CAD build for the part. Positions are in the model's coordinates, mm. Face numbers are marked on the shaded views. A direction names the side the tool comes from. Round coordinates to 2 decimals unless told otherwise and drop trailing zeros. Loops run counter-clockwise (first coordinate to the right, second up) from the corner with the lowest first, then second, coordinate; pieces in that order, holes last. Notation, with made-up numbers: M 44,-4 L 92,-4 A20 ccw 92,21 Z; hole C -7.75,19.5 d2. An arc over 180 degrees is marked long. Use one line per item in the form item = value.
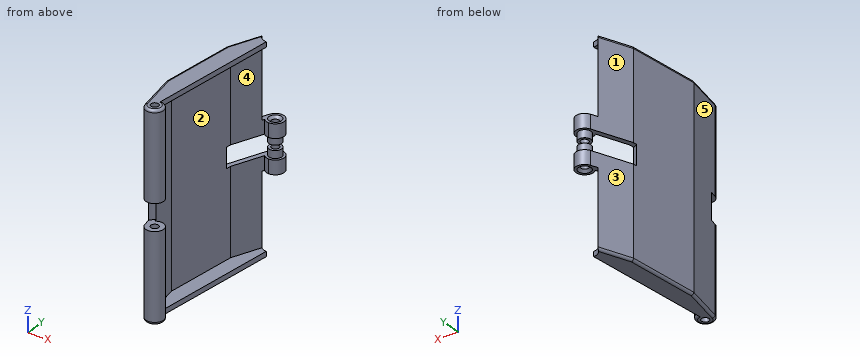
from build123d import *
from build123d.topology import SkipClean

# Parameters (mm, degrees)
CROQUIS2_R              = 1.5
SALIENTE_EXTRUIR1_DEPTH = 40
CORTAR_EXTRUIR8_DEPTH   = 38
CROQUIS21_R             = 4.5
CORTAR_EXTRUIR9_DEPTH   = 30.5
CHAFL_N1_SIZE           = 1
CROQUIS22_R             = 18.418021377
CORTAR_EXTRUIR10_DEPTH  = 4
SALIENTE_EXTRUIR2_START = 3
CROQUIS23_R             = 2.5
CROQUIS23_R_2           = 1.5
SALIENTE_EXTRUIR2_DEPTH = 3
CROQUIS24_R             = 4.5
CORTAR_EXTRUIR11_DEPTH  = 5.2
REDONDEO_CABLE_PLANO_R  = 1


with BuildPart() as part:
    # Croquis2 → Saliente-Extruir1 (new body)
    with BuildSketch(Plane.XY):
        with BuildLine():
            Line((-81.260569926, 30.810305605), (-87.479685276, 15.380704046))
            Line((-87.479685276, 15.380704046), (-90.491189661, -14.467760593))
            Line((-90.491189661, -14.467760593), (-87.479519283, -30.828684819))
            ThreePointArc((-87.479519283, -30.828684819), (-81.463725094, -32.56707429), (-83.686009105, -26.712739874))
            Line((-83.686009105, -26.712739874), (-78.365684691, 26.019547656))
            ThreePointArc((-78.365684691, 26.019547656), (-75.018767914, 31.311988091), (-81.260569926, 30.810305605))
        make_face()
        with Locations((-78.014342512, 29.50186853)):
            Circle(CROQUIS2_R, mode=Mode.SUBTRACT)
        with Locations((-84.037351283, -30.195060749)):
            Circle(CROQUIS2_R, mode=Mode.SUBTRACT)
    extrude(amount=SALIENTE_EXTRUIR1_DEPTH)

    # Croquis20 → Cortar-Extruir8 (cut)
    with BuildSketch(Plane(origin=(0, 0, 0), x_dir=(-1, 0, 0), z_dir=(0, 0, -1))):
        with BuildLine():
            Line((80.58776607, 27.129635154), (85.518345507, 14.896886302))
            Line((85.518345507, 14.896886302), (88.472734145, -14.385476766))
            Line((88.472734145, -14.385476766), (86.085050495, -27.356587931))
            ThreePointArc((86.085050495, -27.356587931), (84.944567837, -26.814682349), (83.686009105, -26.712739874))
            Line((83.686009105, -26.712739874), (78.365684691, 26.019547656))
            ThreePointArc((78.365684691, 26.019547656), (79.578515526, 26.370836307), (80.58776607, 27.129635154))
        make_face()
    extrude(amount=-CORTAR_EXTRUIR8_DEPTH, mode=Mode.SUBTRACT)

    # Croquis21 → Cortar-Extruir9 (cut)
    with BuildSketch(Plane.XY.offset(40)):
        with Locations((-78.014342512, 29.50186853)):
            Circle(CROQUIS21_R)
    extrude(amount=-CORTAR_EXTRUIR9_DEPTH, mode=Mode.SUBTRACT)

    # Chaflán1
    chafl_n1_edges = [part.edges().sort_by_distance(p)[0] for p in [
        (-79.514342512, 29.50186853, 9.5),
    ]]
    chamfer(chafl_n1_edges, length=CHAFL_N1_SIZE)

    # Croquis22 → Cortar-Extruir10 (cut)
    with BuildSketch(Plane(origin=(0, 0, 0), x_dir=(-1, 0, 0), z_dir=(0, 0, -1))):
        with Locations((78.014342512, 29.50186853)):
            Circle(CROQUIS22_R)
    extrude(amount=-CORTAR_EXTRUIR10_DEPTH, mode=Mode.SUBTRACT)

    # Croquis23 → Saliente-Extruir2 (add)
    with SkipClean():  # the faces are left unmerged after this step: merging them gives an invalid solid
        with BuildSketch(Plane(origin=(0, 0, 4), x_dir=(-1, 0, 0), z_dir=(0, 0, -1)).offset(SALIENTE_EXTRUIR2_START)):
            with Locations((78.014342512, 29.50186853)):
                Circle(CROQUIS23_R)
            with Locations((78.014342512, 29.50186853)):
                Circle(CROQUIS23_R_2, mode=Mode.SUBTRACT)
        extrude(amount=-SALIENTE_EXTRUIR2_DEPTH)

    # Croquis24 → Cortar-Extruir11 (cut)
    with SkipClean():  # the faces are left unmerged after this step: merging them gives an invalid solid
        with BuildSketch(Plane(origin=(0, 0, 0), x_dir=(-1, 0, 0), z_dir=(0, 0, -1))):
            with Locations((84.037351283, -30.195060749)):
                Circle(CROQUIS24_R)
        extrude(amount=-CORTAR_EXTRUIR11_DEPTH, mode=Mode.SUBTRACT)

    # Simetría1: part across plane


with BuildPart() as part_1:
    with SkipClean():  # the faces are left unmerged after this step: merging them gives an invalid solid
        add(part.part)
        add(part.part.mirror(Plane(origin=(-78.014342512, 29.50186853, 0), x_dir=(1, 0, 0), z_dir=(0, 0, -1))))

    # Redondeo Cable plano
    redondeo_cable_plano_edges = [part_1.edges().sort_by_distance(p)[0] for p in [
        (-81.463725094, -32.56707429, -40),
        (-84.898816017, 21.783830873, -40),
        (-88.985437468, 0.456471727, -40),
        (-88.985354472, -22.648222706, -40),
        (-88.985437468, 0.456471727, 40),
        (-88.985354472, -22.648222706, 40),
        (-81.463725094, -32.56707429, 40),
        (-84.898816017, 21.783830873, 40),
    ]]
    fillet(redondeo_cable_plano_edges, radius=REDONDEO_CABLE_PLANO_R)


solid = part_1.part
1. Cut at A-A on z = -10.5. Write the cut outline in (x, y), and give its area (3 significant figures).
Completed:
outline = M -90.49,-14.47 L -87.48,-30.83 A3.5 ccw long -86.09,-27.36 L -88.47,-14.39 L -85.52,14.9 L -80.99,26.13 A4.5 cw -82.32,28.19 L -87.48,15.38 Z; hole C -84.04,-30.2 d3
area = 145 mm2
2. Tool access for the marked faces 1 and 2: list every direction of +Z, -Z, +X, -X, +Y, -Y with a clear straight run to the whole face (end or side of a thin tool).
Completed:
face_1 = +Z, -Z, -X, +Y
face_2 = +X
3. Probe line 1 along Z through (x, y) = (-82.5, 6); line 2 along Z through (x, y) = (-82.5, -29.5); line 3 along Y through (x, z) = (-83.25, -29.5). List the from-to ranges inside material, lowest first. Write a range as from..to.
Completed:
line_1 = -40..-38, 38..40
line_2 = -40..-5.2, 5.2..40
line_3 = -33.61..-31.47, -28.92..-26.78, 20.52..25.87
4. Drop flat-ended pins along their axis: P1, Ø3, axis at y = -12, z = -20, coming from the -X side; P2, Ø3.5, axis at x = -78.01, y = 29.5, coming from the +Z side; P3, Ø1, axis at y = -26, z = -15, coming from the +X side. Give the stop position or say it passes through.
Completed:
P1 = -90.39
P2 = 8.75
P3 = -86.24
5. Pull direction Y, two halves, no side cores. Call the marked faces 3, 4 and 5: +Y half, -Y half, draft (parallel to the pull), parting line (faces both ways), or undercut.
Completed:
face_3 = +Y half
face_4 = undercut
face_5 = -Y half
